For this review, use the dimensioned drawing (mm, ordinates from the lowest corner) and the shaded views. A direction names the side the tool comes from. Round coordinates to 2 decimals unless told otherwise and drop trailing zeros. Write each loop counter-clockwise with the first axis right and the second up, starting at its lowest first coordinate (ties: lowest second). Pieces come first, ordered by that corner, then holes.
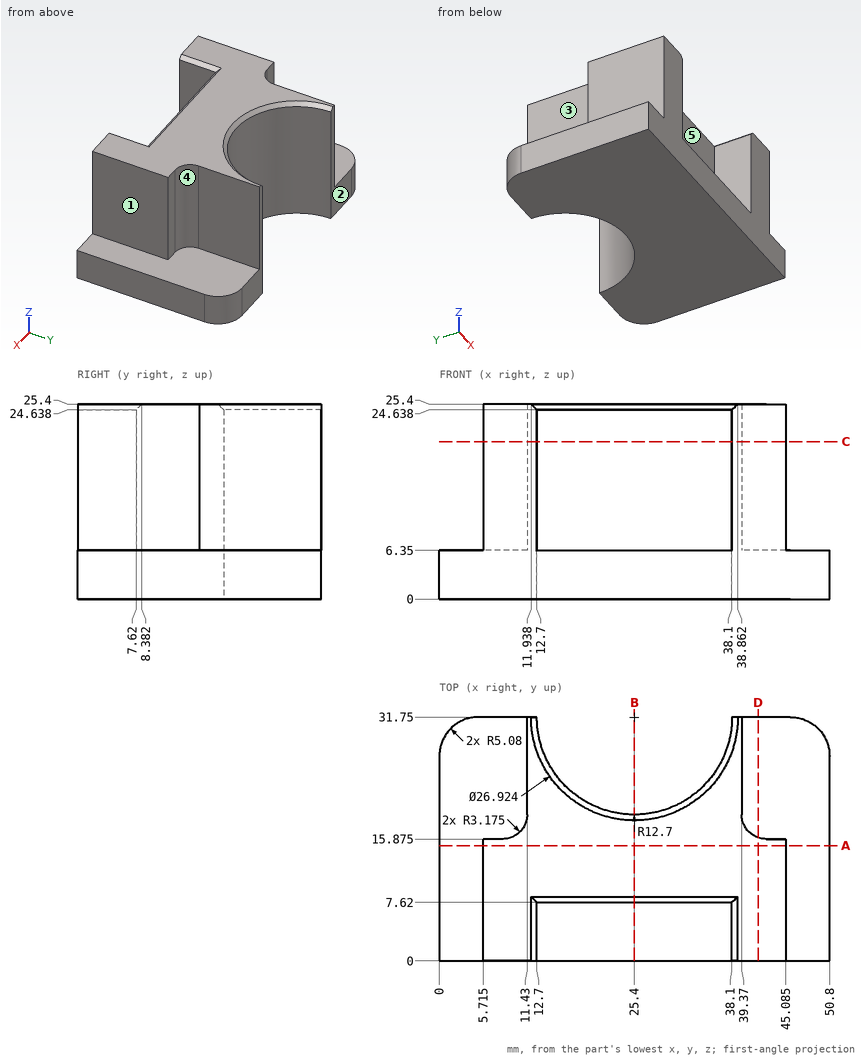
1) For line 1 along X through (y, z) = (4, 9) (3 decimals); line 2 along Y through (x, z) = (7, 22) (3 decimals); line 3 along X through (y, z) = (14, 7) (3 decimals), list the stretches that pass through material, from the lowest coordinate up.
2) Add section A-A on y = 15. State the section outline as (x, z) points (3 decimals), and give its area (3 significant figures).
3) Add section C-C on z = 20.5. State the section outline as (x, y) points (3 decimals).
4) Add section D-D on x = 41.5. State the section outline as (y, z) points, and give its area (3 significant figures).
5) For the marked faces 1, 2, 3, 4 and 5, list the 3-axis set-ups (+Z, -Z, +X, -X, +Y, -Y) from which the entire face can be reached by the end or side of a thin tool; tool diameter is ignored.
6) Add section B-B on x = 25.4. State the section outline as (y, z) points.
7) For P1, Ø2.5, axis at y = 3.5, z = 12.5, coming from the +X side (3 decimals); P2, Ø3, axis at x = 7, z = 20, coming from the +Y side; P3, Ø3, axis at x = 19.5, z = 13.5, coming from the -Y side, all flat-tipped, find the tip position at first contact; note any pin that passes through.
Computed:
1. line 1: x = 5.715 to 12.7, 38.1 to 45.085
1. line 2: y = 0 to 15.875
1. line 3: x = 5.715 to 45.085
2. outline: (0, 0) - (50.8, 0) - (50.8, 6.35) - (45.085, 6.35) - (45.085, 25.4) - (5.715, 25.4) - (5.715, 6.35) - (0, 6.35) - close
2. area: 1,070 mm2
3. outline: (5.715, 0) - (12.7, 0) - (12.7, 7.62) - (38.1, 7.62) - (38.1, 0) - (45.085, 0) - (45.085, 15.875) - (42.545, 15.875) arc R3.175 cw to (39.37, 19.05) - (39.37, 31.75) - (38.1, 31.75) arc R12.7 cw to (12.7, 31.75) - (11.43, 31.75) - (11.43, 19.05) arc R3.175 cw to (8.255, 15.875) - (5.715, 15.875) - close
4. outline: (0, 0) - (31.75, 0) - (31.75, 6.35) - (16.05, 6.35) - (16.05, 25.4) - (0, 25.4) - close
4. area: 507 mm2
5. face 1: +Z, +X, +Y, -Y
5. face 2: +Z, -Z, +X, -X, +Y
5. face 3: +Z, -X, +Y
5. face 4: +Z, +X, +Y
5. face 5: +Z, -Y
6. outline: (0, 0) - (19.05, 0) - (19.05, 24.64) - (18.29, 25.4) - (8.38, 25.4) - (7.62, 24.64) - (7.62, 6.35) - (0, 6.35) - close
7. P1: stops at x = 45.085
7. P2: stops at y = 15.88
7. P3: stops at y = 7.62
